Here's how the part is built. I have some questions about the finished solid (model axes, mm). A direction names the side the tool comes from. Round coordinates to 2 decimals unless told otherwise and drop trailing zeros. Order: outer loops, then holes, each group sorted by start corner. A loop starts at its lowest first (then second) coordinate and runs counter-clockwise, first axis right, second up. Notation, with made-up numbers: (-34, 83) -> (-1, 83) arc R27 cw to (-1, 122) -> close; hole circle Ø3 at (66.25, 82). An arc over 180 degrees is marked (long way). Answer in a Markdown table with one row per item.
```python
from build123d import *

# Parameters (mm, degrees)
SKETCH_1_W          = 50
SKETCH_1_H          = 47
EXTRUDE_1_DEPTH     = 12
SKETCH_2_W          = 50
SKETCH_2_H          = 10
CUT_EXTRUDE_1_DEPTH = 2
SKETCH_3_R          = 2.25
CUT_EXTRUDE_2_DEPTH = 70.663476801
SKETCH_4_W          = 5
SKETCH_4_H          = 37
CUT_EXTRUDE_3_DEPTH = 70.663476801
SKETCH_5_R          = 2
CUT_EXTRUDE_4_DEPTH = 10
CUT_EXTRUDE_START   = -10
SKETCH_6_R          = 2
CUT_EXTRUDE_5_DEPTH = 10
SKETCH_7_R          = 4
CUT_EXTRUDE_6_DEPTH = 4


with BuildPart() as part:
    # 스케치1 → 보스-돌출1 (new body)
    with BuildSketch(Plane.XY):
        with Locations((25, 23.5)):
            Rectangle(SKETCH_1_W, SKETCH_1_H)
    extrude(amount=EXTRUDE_1_DEPTH)

    # 스케치2 → 컷-돌출1 (cut)
    with BuildSketch(Plane(origin=(0, 0, 0), x_dir=(-1, 0, 0), z_dir=(0, 0, -1))):
        with Locations((-25, 42)):
            Rectangle(SKETCH_2_W, SKETCH_2_H)
    extrude(amount=-CUT_EXTRUDE_1_DEPTH, mode=Mode.SUBTRACT)

    # 스케치3 → 컷-돌출2 (cut, through all)
    with BuildSketch(Plane.XY.offset(12)):
        with Locations((25, 42)):
            Circle(SKETCH_3_R)
        with Locations((40, 42)):
            Circle(SKETCH_3_R)
        with Locations((10, 42)):
            Circle(SKETCH_3_R)
    extrude(amount=-CUT_EXTRUDE_2_DEPTH, mode=Mode.SUBTRACT)

    # 스케치4 → 컷-돌출3 (cut, through all)
    with BuildSketch(Plane.XY.offset(12)):
        with Locations((2.5, 18.5)):
            Rectangle(SKETCH_4_W, SKETCH_4_H)
        with Locations((47.5, 18.5)):
            Rectangle(SKETCH_4_W, SKETCH_4_H)
    extrude(amount=-CUT_EXTRUDE_3_DEPTH, mode=Mode.SUBTRACT)

    # 스케치5 → 컷-돌출4 (cut)
    with BuildSketch(Plane(origin=(45, 0, 0), x_dir=(0, 0, -1), z_dir=(1, 0, 0))):
        with Locations((-6, 29.5)):
            Circle(SKETCH_5_R)
        with Locations((-6, 18.5)):
            Circle(SKETCH_5_R)
        with Locations((-6, 7.5)):
            Circle(SKETCH_5_R)
    extrude(amount=-CUT_EXTRUDE_4_DEPTH, mode=Mode.SUBTRACT)

    # 스케치6 → 컷-돌출5 (cut)
    with BuildSketch(Plane.ZY.offset(-5).offset(CUT_EXTRUDE_START)):
        with Locations(Location((6, 29.5, 0), (0, 0, 180))):
            Circle(SKETCH_6_R)
        with Locations(Location((6, 18.5, 0), (0, 0, 180))):
            Circle(SKETCH_6_R)
        with Locations(Location((6, 7.5, 0), (0, 0, 180))):
            Circle(SKETCH_6_R)
    extrude(amount=CUT_EXTRUDE_5_DEPTH, mode=Mode.SUBTRACT)

    # 스케치7 → 컷-돌출6 (cut)
    with BuildSketch(Plane.XY.offset(12)):
        with Locations((10, 42)):
            Circle(SKETCH_7_R)
        with Locations((25, 42)):
            Circle(SKETCH_7_R)
        with Locations((40, 42)):
            Circle(SKETCH_7_R)
    extrude(amount=-CUT_EXTRUDE_6_DEPTH, mode=Mode.SUBTRACT)


solid = part.part
```
1. For faces 1 (the face through (10.07, 6.148, 7.474)), 2 (the face through (35, 8, 6)), 3 (the face through (37.05, 44.7, 10.03)), which set-ups out of +Z, -Z, +X, -X, +Y, -Y let a thin tool reach every point of the face, with its end or its side?
Numbers:
| item | result |
|---|---|
| face 1 | -X |
| face 2 | +X |
| face 3 | +Z |
2. Suppose I cut it at C-C on x = 25. Write out the boundary of the cut face in (y, z), then the cut area to 3 significant figures.
Numbers:
| item | result |
|---|---|
| outline | (0, 0) -> (37, 0) -> (37, 2) -> (39.75, 2) -> (39.75, 8) -> (38, 8) -> (38, 12) -> (0, 12) -> close; (44.25, 2) -> (47, 2) -> (47, 12) -> (46, 12) -> (46, 8) -> (44.25, 8) -> close |
| area | 485 mm2 |
3. Please list where these lines run through material, in increasing order: line 1 along Y through (x, z) = (7.5, 6); line 2 along Y through (x, z) = (10, 5.1); line 3 along X through (y, z) = (3.5, 8.5).
Numbers:
| item | result |
|---|---|
| line 1 | y = 0 to 5.5, 9.5 to 16.5, 20.5 to 27.5, 31.5 to 47 |
| line 2 | y = 0 to 5.71, 9.29 to 16.71, 20.29 to 27.71, 31.29 to 39.75, 44.25 to 47 |
| line 3 | x = 5 to 45 |
4. We'd pull the mould along X, two halves only. Please class faces 4 (the face through (35, 30, 6)), 5 (the face through (15, 7, 6)), 6 (the face through (25, 0, 6)), 7 (the face through (9.71, 44.23, 5.04)): released by +X, released by -X, zero draft, split by the parting line, or undercut.
Numbers:
| item | result |
|---|---|
| face 4 | released by +X |
| face 5 | released by -X |
| face 6 | zero draft |
| face 7 | undercut |
5. Suppose I cut it at D-D on y = 29.5. Write out the boundary of the cut face in (x, z), then the cut area to 3 significant figures.
Numbers:
| item | result |
|---|---|
| outline | (5, 0) -> (45, 0) -> (45, 4) -> (35, 4) -> (35, 8) -> (45, 8) -> (45, 12) -> (5, 12) -> (5, 8) -> (15, 8) -> (15, 4) -> (5, 4) -> close |
| area | 400 mm2 |
6. Suppose I cut it at A-A on x = 40. Write out the boundary of the cut face in (y, z), then the cut area to 3 significant figures.
Numbers:
| item | result |
|---|---|
| outline | (0, 0) -> (37, 0) -> (37, 2) -> (39.75, 2) -> (39.75, 8) -> (38, 8) -> (38, 12) -> (0, 12) -> close; (44.25, 2) -> (47, 2) -> (47, 12) -> (46, 12) -> (46, 8) -> (44.25, 8) -> close; hole circle Ø4 at (7.5, 6); hole circle Ø4 at (18.5, 6); hole circle Ø4 at (29.5, 6) |
| area | 447 mm2 |
7. For pin 1 Ø3 at (y, z) = (8, 7) entering from -X; pin 2 Ø2 at (y, z) = (33, 8.5) entering from +X; pin 3 Ø3 at (y, z) = (18.5, 6) entering from -X; pin 4 Ø2.5 at (x, y) = (24.5, 42) entering from +Z, each with a flat end and sliding along its axis, tell me the tip position at first contact or that it passes through.
Numbers:
| item | result |
|---|---|
| pin 1 | stops at x = 5 |
| pin 2 | stops at x = 45 |
| pin 3 | stops at x = 15 |
| pin 4 | passes through |
8. Suppose I cut it at B-B on y = 42. Write out the boundary of the cut face in (x, z), then the cut area to 3 significant figures.
Numbers:
| item | result |
|---|---|
| outline | (0, 2) -> (7.75, 2) -> (7.75, 8) -> (6, 8) -> (6, 12) -> (0, 12) -> close; (12.25, 2) -> (22.75, 2) -> (22.75, 8) -> (21, 8) -> (21, 12) -> (14, 12) -> (14, 8) -> (12.25, 8) -> close; (27.25, 2) -> (37.75, 2) -> (37.75, 8) -> (36, 8) -> (36, 12) -> (29, 12) -> (29, 8) -> (27.25, 8) -> close; (42.25, 2) -> (50, 2) -> (50, 12) -> (44, 12) -> (44, 8) -> (42.25, 8) -> close |
| area | 323 mm2 |
